Geometry: see drawing. Coordinates: mm, zero at the bounding-box minimum. Give positions to 0.01 mm unless a question says otherwise; leave off trailing zeros. Loops run counter-clockwise (first coordinate to the right, second up) from the corner with the lowest first, then second, coordinate; pieces in that order, holes last. Notation, with made-up numbers: (54.25, 76.5) -> (102.25, 76.5) arc R24 ccw to (102.25, 93.5) -> close; hole circle Ø10 at (3, -9). An arc over 180 degrees is marked (long way). Return JSON: item names as keys, results as strings. Group by question number.
(1) Draft query along Y for the marked faces 1, 2 and 3. Return one class per face: released by +Y, released by -Y, zero draft, split by the parting line, or undercut.
(2) Ray query, line 1 (Y direction, x = 6, z = 12); line 2 (Z direction, x = 6.75, y = 9.25); line 3 (Z direction, x = 6.75, y = 0.75). Return the intervals inside material, ascending. Write a range as from..to.
(3) Cut plane C-C on z = 16.5. Return loops of the section in (x, y).
(4) Cut plane A-A on y = 6. Return loops of the section in (x, z) (3 decimals).
(5) Cut plane D-D on x = 1.75. Return loops of the section in (y, z), then the cut area to 3 significant figures.
(6) Pin query (flat end, axial travel): pin 1 (4 mm diameter, centred on x = 7, z = 33, fed in from +Y) (3 decimals); pin 2 (1.5 mm diameter, centred on x = 9.5, y = 9.5, fed in from +Z); pin 3 (1 mm diameter, centred on x = 6, y = 2, fed in from -Z). Return the tip coordinate at first contact, or that it passes through.
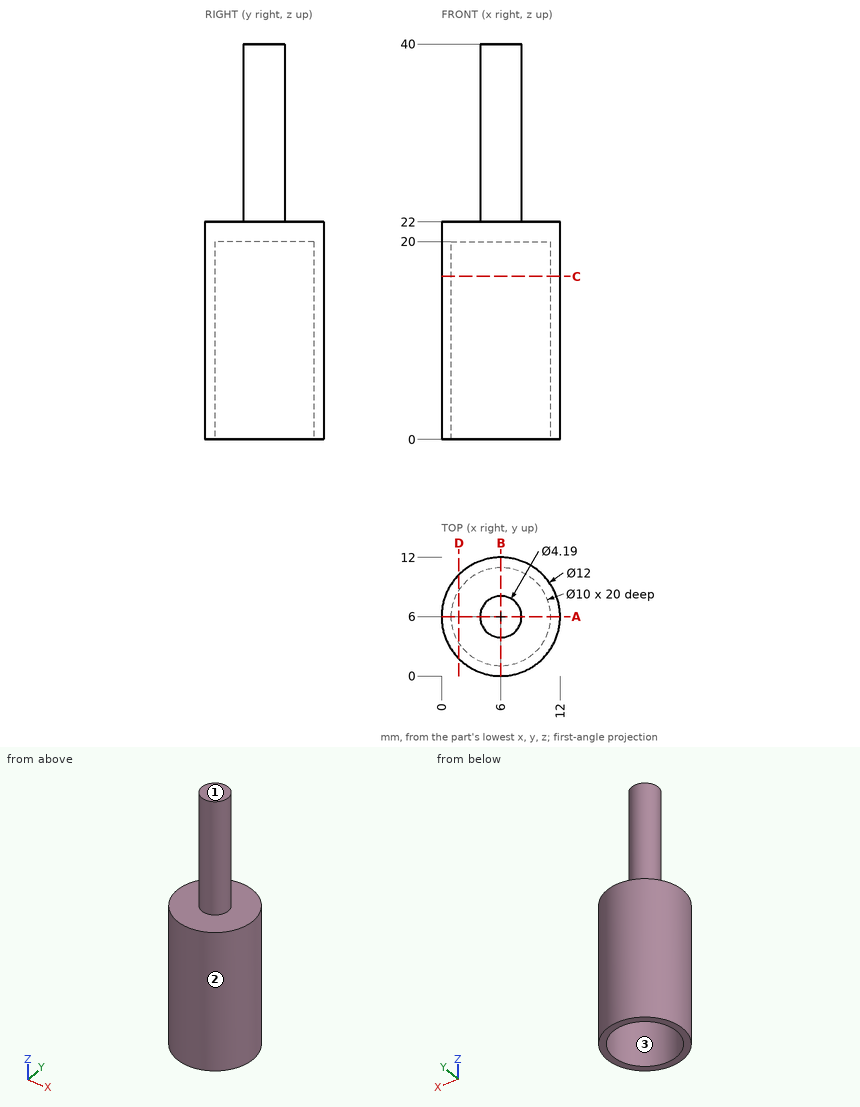
Answers:
{
 "1": {"face 1": "zero draft", "face 2": "split by the parting line", "face 3": "undercut"},
 "2": {"line 1": "0..1, 11..12", "line 2": "20..22", "line 3": "0..22"},
 "3": {"outline": "circle Ø12 at (6, 6); hole circle Ø10 at (6, 6)"},
 "4": {"outline": "(0, 0) -> (1, 0) -> (1, 20) -> (11, 20) -> (11, 0) -> (12, 0) -> (12, 22) -> (8.095, 22) -> (8.095, 40) -> (3.905, 40) -> (3.905, 22) -> (0, 22) -> close"},
 "5": {"outline": "(1.76, 0) -> (3.37, 0) -> (3.37, 20) -> (8.63, 20) -> (8.63, 0) -> (10.24, 0) -> (10.24, 22) -> (1.76, 22) -> close", "area": "81.0 mm²"},
 "6": {"pin 1": "y = 8.095", "pin 2": "z = 22", "pin 3": "z = 20"}
}
